Job drawing, mm, ordinate dimensions from the low corner. One solid piece. A direction names the side the tool comes from. Give positions to 0.01 mm unless a question says otherwise; leave off trailing zeros. Write each loop counter-clockwise with the first axis right and the second up, starting at its lowest first coordinate (ties: lowest second). Pieces come first, ordered by that corner, then holes. Notation, with made-up numbers: (13, -23.75) - (61, -23.75) arc R30 ccw to (61, 12.25) - close; hole circle Ø2 at (41.25, 68). An arc over 180 degrees is marked (long way). Put each result on its own line as item: value. Start each with the question number.
1. Cut at B-B on x = 17. List the corners of the cut face in (y, z) (3 decimals), and give its area (3 significant figures).
2. Cut at C-C on y = 21. List the corners of the cut face in (x, z).
3. Cut at D-D on x = 71. List the corners of the cut face in (y, z) (3 decimals).
4. Drop flat-ended pins along their axis: pin 1 (7 mm diameter, centred on x = 69.5, z = 42.5, fed in from +Y); pin 2 (6 mm diameter, centred on x = 57, y = 22.5, fed in from -Z); pin 3 (9.5 mm diameter, centred on x = 37.5, z = 45.5, fed in from -Y). Give the stop position or say it passes through.
5. Cut at A-A on z = 45.5. List the corners of the cut face in (x, y).
6. Mould opens along Y. For the marked faces 1, 2, 3 and 4 say: +Y half, -Y half, draft (parallel to the pull), parting line (faces both ways), or undercut.
7. Tool access for the marked faces 5, 6 and 7: list every direction of +Z, -Z, +X, -X, +Y, -Y with a clear straight run to the whole face (end or side of a thin tool).
8. Wall check: line 1 (Y direction, x = 17, z = 16.2); line 2 (Y direction, x = 17, z = 19.4); line 3 (Z direction, x = 48, y = 5). Give the ranges that are in metal, low to high.
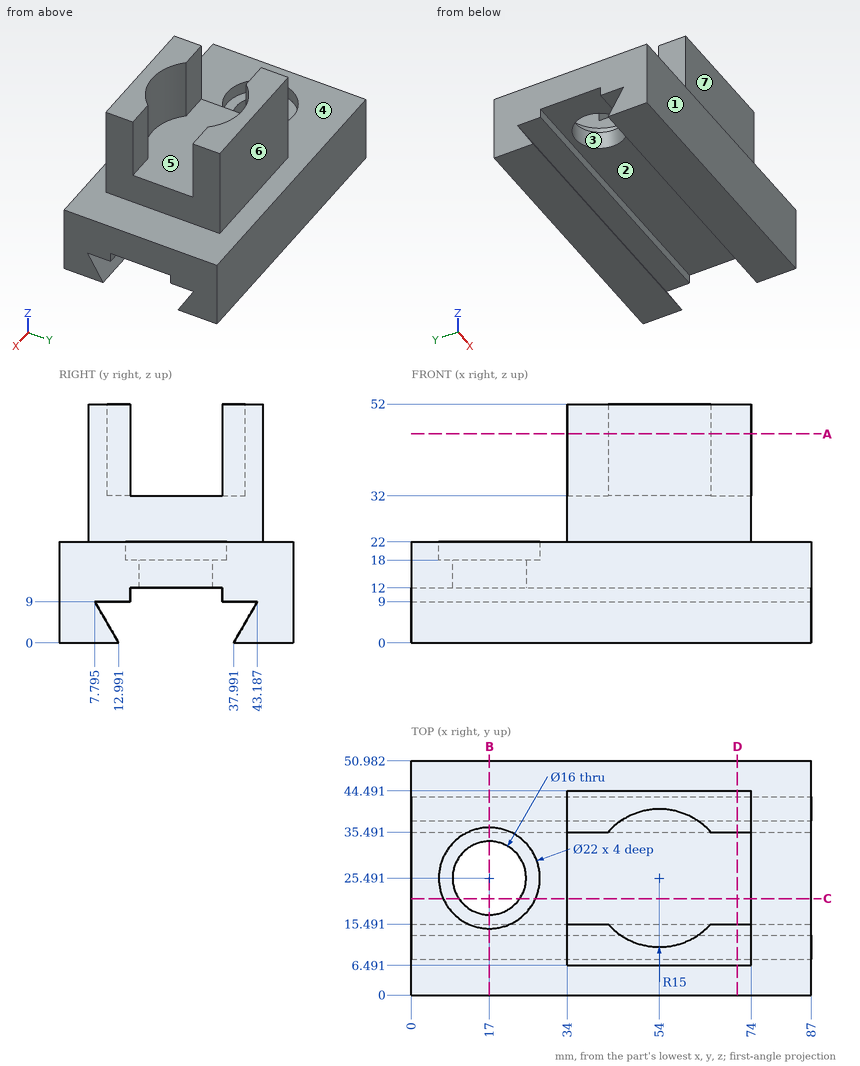
Report:
1. outline: (0, 0) - (12.991, 0) - (7.795, 9) - (15.491, 9) - (15.491, 12) - (17.491, 12) - (17.491, 18) - (14.491, 18) - (14.491, 22) - (0, 22) - close; (33.491, 12) - (35.491, 12) - (35.491, 9) - (43.187, 9) - (37.991, 0) - (50.982, 0) - (50.982, 22) - (36.491, 22) - (36.491, 18) - (33.491, 18) - close
1. area: 606 mm²
2. outline: (0, 12) - (10.38, 12) - (10.38, 18) - (6.96, 18) - (6.96, 22) - (0, 22) - close; (23.62, 12) - (87, 12) - (87, 22) - (74, 22) - (74, 32) - (34, 32) - (34, 22) - (27.04, 22) - (27.04, 18) - (23.62, 18) - close
3. outline: (0, 0) - (12.991, 0) - (7.795, 9) - (15.491, 9) - (15.491, 12) - (35.491, 12) - (35.491, 9) - (43.187, 9) - (37.991, 0) - (50.982, 0) - (50.982, 22) - (44.491, 22) - (44.491, 52) - (35.491, 52) - (35.491, 32) - (15.491, 32) - (15.491, 52) - (6.491, 52) - (6.491, 22) - (0, 22) - close
4. pin 1: stops at y = 44.49
4. pin 2: stops at z = 12
4. pin 3: stops at y = 6.49
5. outline: (34, 6.49) - (74, 6.49) - (74, 15.49) - (65.18, 15.49) arc R15 cw to (42.82, 15.49) - (34, 15.49) - close; (34, 35.49) - (42.82, 35.49) arc R15 cw to (65.18, 35.49) - (74, 35.49) - (74, 44.49) - (34, 44.49) - close
6. face 1: -Y half
6. face 2: undercut
6. face 3: undercut
6. face 4: draft
7. face 5: +Z
7. face 6: +Z, +X, -X, +Y
7. face 7: +Z, +X, -X, -Y
8. line 1: y = 0 to 17.49, 33.49 to 50.98
8. line 2: y = 0 to 14.49, 36.49 to 50.98
8. line 3: z = 0 to 22
